Verification items for the finished model (mm, model axes). Face numbers are marked on the shaded views. A direction names the side the tool comes from. Coordinates: 2 decimals unless noted, no trailing zeros. Order: outer loops, then holes, each group sorted by start corner. A loop starts at its lowest first (then second) coordinate and runs counter-clockwise, first axis right, second up. Notation, with made-up numbers: M -11.75,-33.75 L 31.25,-33.75 A15 cw 31.25,-6.75 Z; hole C 79.25,-35.75 d2. An arc over 180 degrees is marked long. Return JSON: item names as keys, results as strings. Group by question number.
1. Section check A-A, the plane z = 0. Record the cut outline in (x, y).
2. Gauge pin test, flat ends, axial feed: pin 1 (1 mm diameter, centred on x = -0.5, y = -88.5, fed in from +Z); pin 2 (5 mm diameter, centred on x = 0, y = -85.5, fed in from +Z); pin 3 (2 mm diameter, centred on y = -72.5, z = -2.5, fed in from -X); pin 4 (5 mm diameter, centred on y = -45.5, z = -2, fed in from +X). Record the tip position at first contact, or that the pin passes through.
3. Section check B-B, the plane y = -21.5. Record the cut outline in (x, z) (1 decimal), plus the area to 3 significant figures.
4. Material ranges on line 1 along X through (y, z) = (-88.9, 1.5) (3 decimals); line 2 along X through (y, z) = (-22, -4); line 3 along X through (y, z) = (-88.9, 2.9) (3 decimals), recorded low to high.
5. Set-up check for the marked faces 1 and 2: record each of +Z, -Z, +X, -X, +Y, -Y from which the full face is reachable in a straight line by a thin tool's end or side.
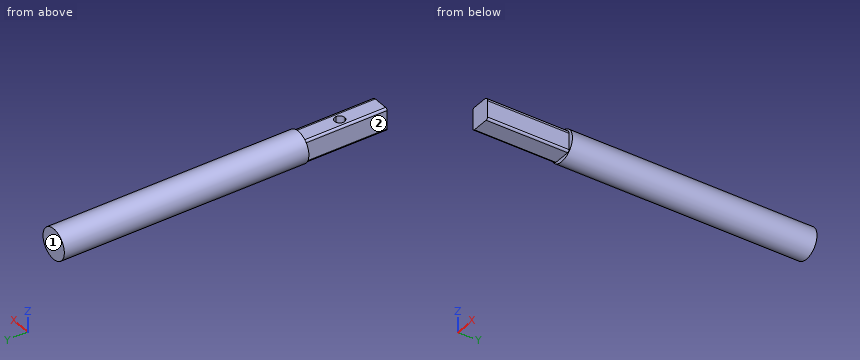
```python
from build123d import *

# Parameters (mm, degrees)
F0_R     = 4.7625
F1_DEPTH = 101.6
F2_R     = 4.7625
F3_DEPTH = 25.4
F5_DEPTH = 2.54


with BuildPart() as f1:
    # F0 (on Front) → F1 (new body)
    with BuildSketch(Plane.XZ):
        Circle(F0_R)
    extrude(amount=F1_DEPTH)

    # F2 (on face) → F3 (cut)
    with BuildSketch(Plane.XZ.offset(101.6)):
        Circle(F2_R)
        with BuildLine():
            ThreePointArc((-3.239123, 2.856345), (-3.053136, 3.305358), (-2.604123, 3.491345))
            Line((-2.604123, 3.491345), (1.969123, 3.491345))
            ThreePointArc((1.969123, 3.491345), (2.867149, 3.11937), (3.239123, 2.221345))
            Line((3.239123, 2.221345), (3.239123, -2.856345))
            ThreePointArc((3.239123, -2.856345), (3.053136, -3.305358), (2.604123, -3.491345))
            Line((2.604123, -3.491345), (-2.604123, -3.491345))
            ThreePointArc((-2.604123, -3.491345), (-3.053136, -3.305358), (-3.239123, -2.856345))
            Line((-3.239123, -2.856345), (-3.239123, 2.856345))
        make_face(mode=Mode.SUBTRACT)
    extrude(amount=-F3_DEPTH, mode=Mode.SUBTRACT)

    # F4 (on face) → F5 (cut)
    with BuildSketch(Plane.XY.offset(3.491345)):
        with BuildLine():
            ThreePointArc((-0.3175, -90.4875), (0.805032, -90.022532), (1.27, -88.9))
            ThreePointArc((1.27, -88.9), (-1.440032, -87.777468), (-0.3175, -90.4875))
        make_face()
    extrude(amount=-F5_DEPTH, mode=Mode.SUBTRACT)


solid = f1.part
```
Answers follow:
{
 "1": {"outline": "M -4.76,-76.2 L -3.24,-76.2 L -3.24,-101.6 L 3.24,-101.6 L 3.24,-76.2 L 4.76,-76.2 L 4.76,0 L -4.76,0 Z"},
 "2": {"pin 1": "z = 0.95", "pin 2": "z = 3.49", "pin 3": "x = -4.52", "pin 4": "x = 4.76"},
 "3": {"outline": "C 0,0 d9.5", "area": "71.3 mm^2"},
 "4": {"line 1": "-3.239 to -1.905, 1.27 to 3.239", "line 2": "-2.58 to 2.58", "line 3": "-3.238 to -1.905, 1.27 to 3.043"},
 "5": {"face 1": "+Z, -Z, +X, -X, +Y", "face 2": "+Z, -Z, -X, -Y"}
}
